```python
from build123d import *

# Parameters (mm, degrees)
F1_DEPTH = 12.7


with BuildPart() as f1:
    # F0 (on Front) → F1 (new body)
    with BuildSketch(Plane.XZ):
        with BuildLine():
            Line((-30.6719616055, 12.9689474719), (-30.6719616055, 42.5025746226))
            Line((-30.6719616055, 42.5025746226), (-1.1383344548, 42.5025746226))
            ThreePointArc((-1.1383344548, 42.5025746226), (-41.091738146, 70.1370348042), (-52.8531736535, 23.0031139951))
            ThreePointArc((-52.8531736535, 23.0031139951), (-42.8445811442, 15.5941657836), (-30.6719616055, 12.9689474719))
        make_face()
        with BuildLine():
            Line((-1.1383344548, 42.5025746226), (-30.6719616055, 42.5025746226))
            Line((-30.6719616055, 42.5025746226), (-30.6719616055, 12.9689474719))
            ThreePointArc((-30.6719616055, 12.9689474719), (-9.7885335742, 21.6191465913), (-1.1383344548, 42.5025746226))
        make_face()
        with BuildLine():
            Line((36.1052788794, 42.5025746226), (-1.1383344548, 42.5025746226))
            ThreePointArc((-1.1383344548, 42.5025746226), (-9.7885335742, 21.6191465913), (-30.6719616055, 12.9689474719))
            Line((-30.6719616055, 12.9689474719), (-30.6719616055, -46.2820419996))
            ThreePointArc((-30.6719616055, -46.2820419996), (-30.3101183632, -46.7587404599), (-29.9050042347, -47.1992566308))
            Line((-29.9050042347, -47.1992566308), (6.5738577877, -47.1992566308))
            ThreePointArc((6.5738577877, -47.1992566308), (15.2234107674, -26.3173885188), (36.1052788794, -17.6678355391))
            Line((36.1052788794, -17.6678355391), (36.1052788794, 42.5025746226))
        make_face()
        with BuildLine():
            Line((-30.6719616055, -46.2820419996), (-30.6719616055, 12.9689474719))
            ThreePointArc((-30.6719616055, 12.9689474719), (-42.8445811442, 15.5941657836), (-52.8531736535, 23.0031139951))
            Line((-52.8531736535, 23.0031139951), (-31.4936938255, -44.5985173325))
            ThreePointArc((-31.4936938255, -44.5985173325), (-31.1452529672, -45.4707495734), (-30.6719616055, -46.2820419996))
        make_face()
        with BuildLine():
            ThreePointArc((-29.9050042347, -47.1992566308), (-30.3101183632, -46.7587404599), (-30.6719616055, -46.2820419996))
            Line((-30.6719616055, -46.2820419996), (-30.6719616055, -47.1992566308))
            Line((-30.6719616055, -47.1992566308), (-29.9050042347, -47.1992566308))
        make_face()
        with BuildLine():
            ThreePointArc((65.6366999711, -47.1992566308), (56.9871469914, -26.3173885188), (36.1052788794, -17.6678355391))
            Line((36.1052788794, -17.6678355391), (36.1052788794, -47.1992566308))
            Line((36.1052788794, -47.1992566308), (6.5738577877, -47.1992566308))
            ThreePointArc((6.5738577877, -47.1992566308), (10.040761487, -61.0825474799), (19.6274635862, -71.7061216865))
            ThreePointArc((19.6274635862, -71.7061216865), (49.9885697285, -73.2637740232), (65.6366999711, -47.1992566308))
        make_face()
        with BuildLine():
            Line((36.1052788794, -47.1992566308), (36.1052788794, -17.6678355391))
            ThreePointArc((36.1052788794, -17.6678355391), (15.2234107674, -26.3173885188), (6.5738577877, -47.1992566308))
            Line((6.5738577877, -47.1992566308), (36.1052788794, -47.1992566308))
        make_face()
        with BuildLine():
            Line((6.5738577877, -47.1992566308), (-29.9050042347, -47.1992566308))
            ThreePointArc((-29.9050042347, -47.1992566308), (-29.1114169079, -47.865539345), (-28.2200330558, -48.3938842407))
            Line((-28.2200330558, -48.3938842407), (19.6274635862, -71.7061216865))
            ThreePointArc((19.6274635862, -71.7061216865), (10.040761487, -61.0825474799), (6.5738577877, -47.1992566308))
        make_face()
    extrude(amount=F1_DEPTH)


solid = f1.part
```
Input: part model. Units: mm. Frame: model coordinates. A direction names the side the tool comes from. Coordinates: 2 decimals unless noted, no trailing zeros. Loops run counter-clockwise (first coordinate to the right, second up) from the corner with the lowest first, then second, coordinate; pieces in that order, holes last. Notation, with made-up numbers: M -17,-37 L 31,-37 A17 ccw 31,-16 Z; hole C 15.5,75 d8. An arc over 180 degrees is marked long. Answer in a Markdown table with one row per item.
1. First-contact query: pin 1 (2 mm diameter, centred on y = -11.5, z = -60, fed in from +X); pin 2 (6 mm diameter, centred on x = -14, y = -4.5, fed in from -Z); pin 3 (1.5 mm diameter, centred on x = -19.5, y = -8, fed in from +Z). Flat tips, straight axial feed; report the tip coordinate or a pass-through.
Response:
| item | result |
|---|---|
| pin 1 | stops at x = 63.18 |
| pin 2 | stops at z = -56.78 |
| pin 3 | stops at z = 70.14 |
2. Section B-B, the plane z = 47. Output: boundary loops of the cut face in (x, y), then the cut area to 3 significant figures.
Response:
| item | result |
|---|---|
| outline | M -59.86,-12.7 L -1.48,-12.7 L -1.48,0 L -59.86,0 Z |
| area | 741 mm2 |
3. Section C-C, the plane x = -42. Output: boundary loops of the cut face in (y, z).
Response:
| item | result |
|---|---|
| outline | M -12.7,-11.35 L 0,-11.35 L 0,69.78 L -12.7,69.78 Z |
4. Section A-A, the plane y = -9. Output: boundary loops of the cut face in (x, z) (3 decimals).
Response:
| item | result |
|---|---|
| outline | M -52.853,23.003 L -31.494,-44.599 A6.35 ccw -30.672,-46.282 L -30.672,-47.199 L -29.905,-47.199 A6.35 ccw -28.22,-48.394 L 19.627,-71.706 A29.531 ccw long 36.105,-17.668 L 36.105,42.503 L -1.138,42.503 A29.534 ccw long Z |
5. Material intervals for line 1 (Z direction, x = 35.5, y = -7); line 2 (X direction, y = -9.5, z = 63.5); line 3 (Z direction, x = 33.5, y = -5.25), sorted ascending.
Response:
| item | result |
|---|---|
| line 1 | z = -76.72 to 42.5 |
| line 2 | x = -51.44 to -9.9 |
| line 3 | z = -76.62 to 42.5 |
6. Reachability of faces 1 (the flat face through (18, -6, 42.503)), 2 (the flat face through (2, -12.7, -1)) from +Z, -Z, +X, -X, +Y, -Y: full face, straight path, thin tool, end or side. Return the list, or none.
Response:
| item | result |
|---|---|
| face 1 | +Z, +X, +Y, -Y |
| face 2 | +Z, -Z, +X, -X, -Y |
